Work out the finished part from the listing and answer in its coordinate system (mm). A direction names the side the tool comes from. Round coordinates to 2 decimals unless told otherwise and drop trailing zeros. Order: outer loops, then holes, each group sorted by start corner. A loop starts at its lowest first (then second) coordinate and runs counter-clockwise, first axis right, second up. Notation, with made-up numbers: (-18.75, -15.75) - (29.25, -15.75) arc R21 ccw to (29.25, -0.75) - close; hole circle Ø10 at (-35.5, 56.25). An arc over 180 degrees is marked (long way). Answer in a Markdown table with one row per item.
from build123d import *

# Parameters (mm, degrees)
F1_DEPTH  = 20
F2_R      = 3.75
F3_DEPTH  = 4.5
F5_R      = 1.625
F6_DEPTH  = 2
F8_R      = 3
F9_DEPTH  = 7.1339190804
F11_R     = 1.75
F12_DEPTH = 2
F14_R     = 3.75
F15_DEPTH = 12.3627990274


with BuildPart() as f1:
    # F0 (on Front) → F1 (new body, symmetric)
    with BuildSketch(Plane.XZ):
        Polygon((0, 20), (0, 0), (13.8581929877, 14.2597485145), (14.1421356237, 34.1421356237), align=None)
    extrude(amount=F1_DEPTH, both=True)

    # F2 (on Right) → F3 (cut)
    with BuildSketch(Plane.YZ):
        with Locations((10, 10)):
            Circle(F2_R)
        with Locations((-10, 10)):
            Circle(F2_R)
    extrude(amount=F3_DEPTH, mode=Mode.SUBTRACT)

    # F5 (on offset) → F6 (cut)
    with BuildSketch(Plane(origin=(4.5, 0, 0), x_dir=(0, -1, 0), z_dir=(-1, 0, 0))):
        with Locations((-10, 10)):
            Circle(F5_R)
        with Locations((10, 10)):
            Circle(F5_R)
    extrude(amount=-F6_DEPTH, mode=Mode.SUBTRACT)

    # F8 (on offset) → F9 (cut, up to face)
    with BuildSketch(Plane(origin=(6.5, 0, 0), x_dir=(0, -1, 0), z_dir=(-1, 0, 0))):
        with Locations((-10, 10)):
            Circle(F8_R)
        with Locations((10, 10)):
            Circle(F8_R)
    extrude(amount=-F9_DEPTH, mode=Mode.SUBTRACT)

    # F11 (on offset) → F12 (cut)
    with BuildSketch(Plane(origin=(-10, 0, 10), x_dir=(0, -1, 0), z_dir=(-0.7071067812, 0, 0.7071067812))):
        with Locations((-10, 24.1421356237)):
            Circle(F11_R)
        with Locations((10, 24.1421356237)):
            Circle(F11_R)
    extrude(amount=-F12_DEPTH, mode=Mode.SUBTRACT)

    # F14 (on offset) → F15 (cut, up to face)
    with BuildSketch(Plane(origin=(-8.5857864376, 0, 8.5857864376), x_dir=(0, -1, 0), z_dir=(-0.7071067812, 0, 0.7071067812))):
        with Locations((-10, 24.1421356237)):
            Circle(F14_R)
        with Locations((10, 24.1421356237)):
            Circle(F14_R)
    extrude(amount=-F15_DEPTH, mode=Mode.SUBTRACT)


solid = f1.part
1) Find section B-B, the plane y = 10. Give the number of separate pieces and of enclosed holes in the cut face, then the cut area to 3 significant figures.
Filled in:
| item | result |
|---|---|
| separate pieces | 3 |
| enclosed holes | 0 |
| area | 153 mm^2 |
2) Find section D-D, the plane y = 5. Give the vertices of the cut face in (x, z).
Filled in:
| item | result |
|---|---|
| outline | (0, 0) - (13.86, 14.26) - (14.14, 34.14) - (0, 20) - close |
3) Each of these flat-tipped pins is pushed along its axis until it touches: pin 1 (5 mm diameter, centred on x = 9, y = -5, fed in from +Z); pin 2 (4 mm diameter, centred on x = 10, y = -7.5, fed in from +Z); pin 3 (6.5 mm diameter, centred on y = -11.5, z = 11.5, fed in from +X). Where does it stop, or does it pass through?
Filled in:
| item | result |
|---|---|
| pin 1 | stops at z = 31.5 |
| pin 2 | stops at z = 32 |
| pin 3 | stops at x = 13.87 |
4) Which of the six approach directions +Z, -Z, +X, -X, +Y, -Y give full straight-line access (tool end or side, diameter ignored) to faces 1 (the face through (4.5, -8, 9)), 2 (the face through (6.5, 8.7, 8.7)), 3 (the face through (7, -20, 17))?
Filled in:
| item | result |
|---|---|
| face 1 | -X |
| face 2 | +X |
| face 3 | +Z, -Z, +X, -X, -Y |
5) Find section C-C, the plane x = 5. Give the vertices of the cut face in (y, z) (3 decimals), then the cut area to 3 significant figures.
Filled in:
| item | result |
|---|---|
| outline | (-20, 5.145) - (20, 5.145) - (20, 25) - (-20, 25) - close; hole circle Ø3.25 at (-10, 10); hole circle Ø3.25 at (10, 10) |
| area | 778 mm^2 |
6) Find the intervals of material crossed by probe 1 along Y at (x, z) = (9, 10); probe 2 along Z at (x, y) = (5.8, -10) (3 decimals); probe 3 along X at (y, z) = (-18, 10), in increasing order. Write a range as from..to.
Filled in:
| item | result |
|---|---|
| probe 1 | y = -20..-13, -7..7, 13..20 |
| probe 2 | z = 5.968..8.375, 11.625..25.8 |
| probe 3 | x = 0..9.72 |
7) The mould has two halves that part along Z. Classify faces 4 (the face through (7, 20, 17)), 5 (the face through (9, 10, 13)), 6 (the face through (7, 0, 27)): released by +Z, released by -Z, zero draft, split by the parting line, or undercut.
Filled in:
| item | result |
|---|---|
| face 4 | zero draft |
| face 5 | undercut |
| face 6 | released by +Z |
8) Find section A-A, the plane z = 10. Give the vertices of the cut face in (x, y) (3 decimals).
Filled in:
| item | result |
|---|---|
| outline | (0, -20) - (9.718, -20) - (9.718, -13) - (6.5, -13) - (6.5, -11.625) - (4.5, -11.625) - (4.5, -13.75) - (0, -13.75) - close; (0, -6.25) - (4.5, -6.25) - (4.5, -8.375) - (6.5, -8.375) - (6.5, -7) - (9.718, -7) - (9.718, 7) - (6.5, 7) - (6.5, 8.375) - (4.5, 8.375) - (4.5, 6.25) - (0, 6.25) - close; (0, 13.75) - (4.5, 13.75) - (4.5, 11.625) - (6.5, 11.625) - (6.5, 13) - (9.718, 13) - (9.718, 20) - (0, 20) - close |
